Study the drawing (mm; zero at the part's minimum x, y, z) and answer. Coordinates: 2 decimals unless noted, no trailing zeros. Order: outer loops, then holes, each group sorted by start corner. A loop starts at its lowest first (then second) coordinate and runs counter-clockwise, first axis right, second up.
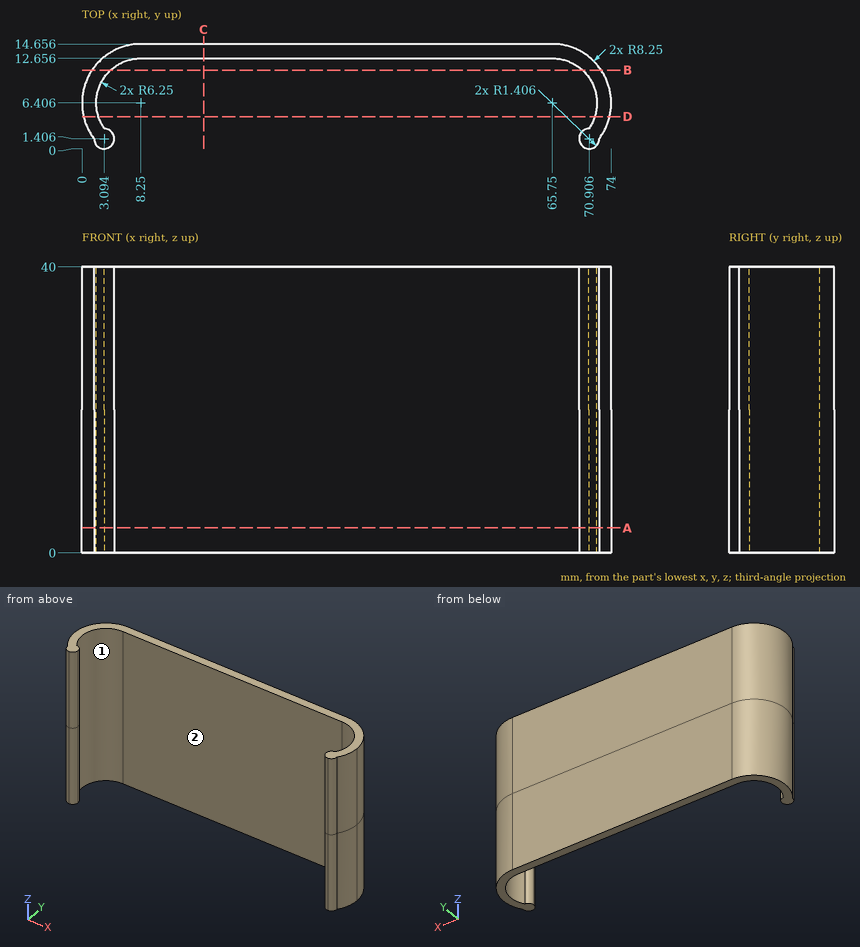
(1) Find section B-B (y = 11). Write down the section's boundary in (x, z).
(2) Find section A-A (z = 3.5). Write down the section's boundary in (x, y).
(3) The mould has two halves that part along X. Classify the marked faces 1 and 2: released by +X, released by -X, zero draft, split by the parting line, or undercut.
(4) Consider line 1 (Y direction, x = 35, z = 24); line 2 (X direction, y = 1, z = 26); line 3 (X direction, y = 7.75, z = 18.5). Determine where each line is inside the solid, lowest interval first.
(5) Find section C-C (x = 17). Write down the section's boundary in (y, z).
(6) Find section D-D (y = 4.5). Write down the section's boundary in (x, z).
(7) Each of these flat-tipped pins is pushed along its axis until it touches: pin 1 Ø3 at (x, y) = (10.5, 9.5) entering from +Z; pin 2 Ø1.5 at (y, z) = (5.5, 7.5) entering from -X; pin 3 Ø1.5 at (y, z) = (2, 23.5) entering from -X. Where does it stop, or does it pass through?
Findings below:
1. outline: (1.4, 0) - (4.01, 0) - (4.01, 40) - (1.4, 40) - close; (69.99, 0) - (72.6, 0) - (72.6, 40) - (69.99, 40) - close
2. outline: (1.69, 1.41) arc R1.41 ccw (long way) to (3.14, 2.81) arc R6.25 cw to (8.25, 12.66) - (65.75, 12.66) arc R6.25 cw to (70.86, 2.81) arc R1.41 ccw (long way) to (72.31, 1.41) arc R8.25 ccw to (65.75, 14.66) - (8.25, 14.66) arc R8.25 ccw to start
3. face 1: undercut
3. face 2: undercut
4. line 1: y = 12.66 to 14.66
4. line 2: x = 1.75 to 4.44, 69.56 to 72.25
4. line 3: x = 0.11 to 2.15, 71.85 to 73.89
5. outline: (12.66, 0) - (14.66, 0) - (14.66, 40) - (12.66, 40) - close
6. outline: (0.22, 0) - (2.3, 0) - (2.3, 40) - (0.22, 40) - close; (71.7, 0) - (73.78, 0) - (73.78, 40) - (71.7, 40) - close
7. pin 1: passes through
7. pin 2: stops at x = 0
7. pin 3: stops at x = 0.85
